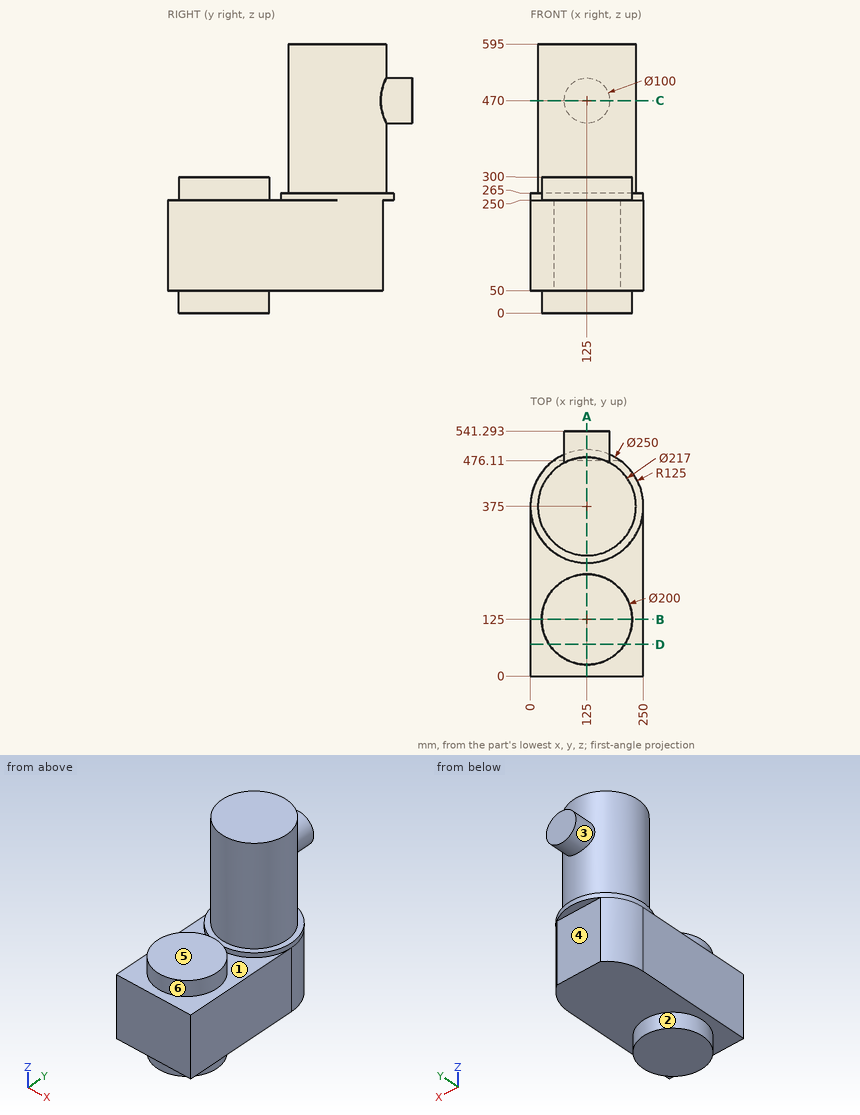
Geometry: see drawing. Coordinates: mm, zero at the bounding-box minimum. A direction names the side the tool comes from. Give positions to 0.01 mm unless a question says otherwise; leave off trailing zeros. Write each loop counter-clockwise with the first axis right and the second up, starting at its lowest first coordinate (ties: lowest second). Pieces come first, ordered by that corner, then holes. Notation, with made-up numbers: M 3,-36.75 L 58,-36.75 A23 cw 58,-11.75 Z; hole C 20.25,10 d6. An arc over 180 degrees is marked long. Return JSON: item names as keys, results as strings. Group by question number.
1) Set-up query: the marked faces 1, 2 and 3. Return all of +Z, -Z, +X, -X, +Y, -Y with unobstructed straight access to the full face (end or side cutting, diameter ignored); none if empty.
2) Draft query along Y for the marked faces 4, 5 and 6. Return one class per face: released by +Y, released by -Y, zero draft, split by the parting line, or undercut.
3) Cut plane B-B, the plane y = 125. Output: boundary loops of the cut face in (x, z).
4) First-contact query: pin 1 Ø1 at (x, z) = (46.5, 134) entering from +Y; pin 2 Ø2 at (x, z) = (143, 118) entering from +Y; pin 3 Ø1 at (x, z) = (197.5, 291) entering from +Y. Flat tips, straight axial feed; report the tip coordinate or a pass-through.
5) Cut plane C-C, the plane z = 470. Output: boundary loops of the cut face in (x, y).
6) Cut plane A-A, the plane x = 125. Output: boundary loops of the cut face in (y, z), then the cut area to 3 significant figures.
7) Cut plane D-D, the plane y = 70. Output: boundary loops of the cut face in (x, z), then the cut area to 3 significant figures.
8) Ray query, L1, parallel to Y at x = 143.5, z = 87.5; L2, parallel to Z at x = 146, y = 232; L3, parallel to Y at x = 105, z = 279. Return the intervals inside material, ascending.
Data:
{
 "1": {"face 1": "+Z", "face 2": "-Z", "face 3": "+Y"},
 "2": {"face 4": "released by +Y", "face 5": "zero draft", "face 6": "undercut"},
 "3": {"outline": "M 0,50 L 25,50 L 25,0 L 225,0 L 225,50 L 250,50 L 250,250 L 225,250 L 225,300 L 25,300 L 25,250 L 0,250 Z"},
 "4": {"pin 1": "stops at y = 472.68", "pin 2": "stops at y = 476.11", "pin 3": "stops at y = 456.17"},
 "5": {"outline": "M 75,471.29 A108.5 ccw long 175,471.29 L 175,541.29 L 75,541.29 Z"},
 "6": {"outline": "M 0,50 L 25,50 L 25,0 L 225,0 L 225,50 L 476.11,50 L 476.11,250 L 500,250 L 500,265 L 483.5,265 L 483.5,420 L 541.29,420 L 541.29,520 L 483.5,520 L 483.5,595 L 266.5,595 L 266.5,265 L 250,265 L 250,250 L 225,250 L 225,300 L 25,300 L 25,250 L 0,250 Z", "area": "196,000 mm²"},
 "7": {"outline": "M 0,50 L 41.48,50 L 41.48,0 L 208.52,0 L 208.52,50 L 250,50 L 250,250 L 208.52,250 L 208.52,300 L 41.48,300 L 41.48,250 L 0,250 Z", "area": "66,700 mm²"},
 "8": {"L1": "y = 0 to 476.11", "L2": "z = 50 to 250", "L3": "y = 27.02 to 222.98, 268.36 to 481.64"}
}
